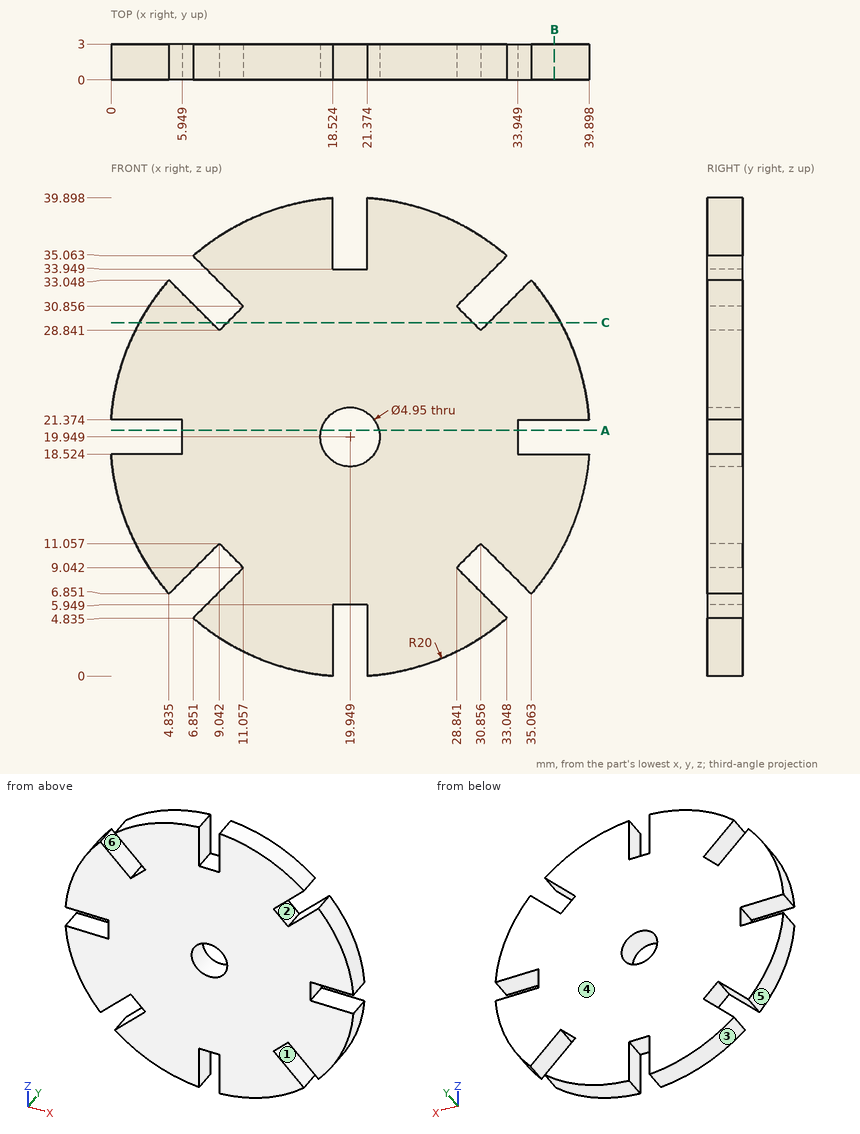
Design review of the part shown in the three views and the two pictorial views. Dimensions are in mm from the part's minimum x, y and z. A direction names the side the tool comes from. Coordinates: 2 decimals unless noted, no trailing zeros. Order: outer loops, then holes, each group sorted by start corner. A loop starts at its lowest first (then second) coordinate and runs counter-clockwise, first axis right, second up. Notation, with made-up numbers: (19.25, 33.25) - (57.25, 33.25) arc R20 ccw to (57.25, 63.25) - close; hole circle Ø1 at (75, -5.75). An arc over 180 degrees is marked (long way). One line per question, with ' | ' between items.
Q1. Consider section B-B, the plane x = 37. Give the boundary of the cut face in (y, z).
Answer key:
outline: (0, 9.5) - (3, 9.5) - (3, 18.52) - (0, 18.52) - close; (0, 21.37) - (3, 21.37) - (3, 30.4) - (0, 30.4) - close
Q2. Consider section C-C, the plane z = 29.5. Give the boundary of the cut face in (x, y) (1 decimal).
Answer key:
outline: (2.4, 0) - (8.4, 0) - (8.4, 3) - (2.4, 3) - close; (9.7, 0) - (30.2, 0) - (30.2, 3) - (9.7, 3) - close; (31.5, 0) - (37.5, 0) - (37.5, 3) - (31.5, 3) - close
Q3. Clearance check with flat-ended pins moving along their axes: pin 1 Ø1.5 at (y, z) = (1, 28.5) entering from -X; pin 2 Ø8 at (x, z) = (19.95, 19.95) entering from -Y; pin 3 Ø1.5 at (x, y) = (3.5, 2) entering from +Z; pin 4 Ø1.4 at (x, y) = (20, 1.5) entering from +Z. State where each tip first meets the part, or that it passes through.
Answer key:
pin 1: stops at x = 1.53 | pin 2: stops at y = 0 | pin 3: stops at z = 32.34 | pin 4: stops at z = 33.95
Q4. Consider section A-A, the plane z = 20.5. Give the boundary of the cut face in (x, y).
Answer key:
outline: (5.95, 0) - (17.54, 0) - (17.54, 3) - (5.95, 3) - close; (22.36, 0) - (33.95, 0) - (33.95, 3) - (22.36, 3) - close
Q5. The part is to be moulded in two halves that separate along Z. For the marked faces 1, 2, 3 and 4, say which applies: +Z half, -Z half, draft (parallel to the pull), parting line (faces both ways), or undercut.
Answer key:
face 1: undercut | face 2: undercut | face 3: -Z half | face 4: draft
Q6. To check wall thickness, follow line 1 along Z through (x, y) = (9.5, 2.85) (1 decimal); line 2 along Z through (x, y) = (10.5, 2.05) (1 decimal); line 3 along X through (y, z) = (0.85, 8) (1 decimal). State the ranges of each line that lie inside material, in increasing order.
Answer key:
line 1: z = 2.9 to 7.5, 10.6 to 29.3, 32.4 to 37 | line 2: z = 2.3 to 8.5, 9.6 to 30.3, 31.4 to 37.6 | line 3: x = 3.9 to 6, 10 to 29.9, 33.9 to 36
Q7. For the marked faces 5 and 6, list the 3-axis set-ups (+Z, -Z, +X, -X, +Y, -Y) from which the entire face can be reached by the end or side of a thin tool; tool diameter is ignored.
Answer key:
face 5: -Z, -X, +Y, -Y | face 6: +Y, -Y
